Check sheet for the modelled part. Datum: model origin and axes. Units: mm. Face numbers are marked on the shaded views. A direction names the side the tool comes from. Give positions to 0.01 mm unless a question says otherwise; leave off trailing zeros. Write each loop counter-clockwise with the first axis right and the second up, starting at its lowest first coordinate (ties: lowest second). Pieces come first, ordered by that corner, then holes. Notation, with made-up numbers: M 19,72.25 L 48,72.25 A25 cw 48,111.25 Z; hole C 14,-39 d3. An arc over 180 degrees is marked long. Write item = value, one per line. Start each with the question number.
1) Sectioned sample at B-B, the plane y = -51. Record the cut outline in (x, z).
2) Draft check along Y on the marked faces 1 and 2. Enter one of: pulls with the +Y half, pulls with the -Y half, needs draft (parallel to the pull), parting line crosses it, or undercut.
3) Sectioned sample at C-C, the plane y = 81. Record the cut outline in (x, z).
4) Gauge pin test, flat ends, axial feed: pin 1 (1 mm diameter, centred on x = -19, y = 30.5, fed in from +Z); pin 2 (12 mm diameter, centred on x = 21, y = -12, fed in from -Z); pin 3 (12 mm diameter, centred on y = -19, z = -71, fed in from +X). Record the tip position at first contact, or that the pin passes through.
5) Sectioned sample at A-A, the plane z = -68.5. Count the separate pieces of the cut face and the enclosed holes in it, then the cut area to 3 significant figures.
6) Set-up check for the marked faces 3 and 4: record each of +Z, -Z, +X, -X, +Y, -Y from which the full face is reachable in a straight line by a thin tool's end or side.
7) Scan lines: L1, parallel to Y at x = 41, z = 67; L2, parallel to Z at x = -11.5, y = 40.5; L3, parallel to Z at x = 9.5, y = -38.5. Record each from-to range of solid material in increasing order.
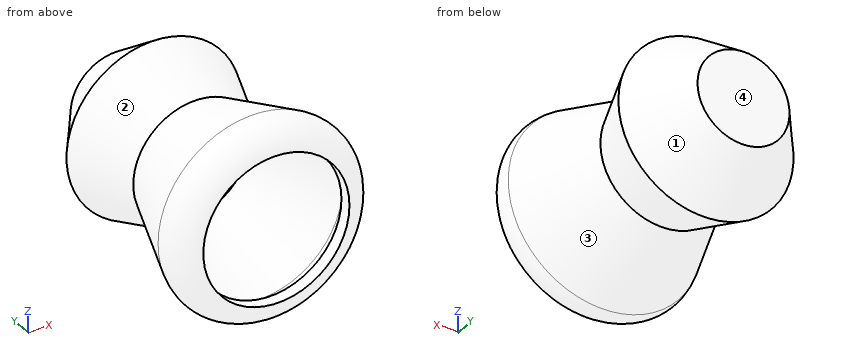
from build123d import *

# Parameters (mm, degrees)
F0_R     = 63.5
F1_DEPTH = 127
F1_TAPER = -20
F2_R     = 25.4
F3_SIZE  = 63.5
F4_T     = -12.7


# Not quite as in the source:
# - a shell that OpenCascade refuses in one call is made with other operations: the cavity is built on its own and cut out


with BuildPart() as f1:
    # F0 (on Front) → F1 (new body, symmetric)
    with BuildSketch(Plane.XZ):
        with Locations((0.2353243763, -0.2353235031)):
            Circle(F0_R)
    extrude(amount=F1_DEPTH, both=True, taper=F1_TAPER)

    # F2
    f2_edges = [f1.edges().sort_by_distance(p)[0] for p in [
        (-109.488895, -127, -0.235324),
    ]]
    fillet(f2_edges, radius=F2_R)

    # F3
    f3_edges = [f1.edges().sort_by_distance(p)[0] for p in [
        (-109.488895, 127, -0.235324),
    ]]
    chamfer(f3_edges, length=F3_SIZE)

    # F4: a shell. OpenCascade refuses it in one call, so the cavity is built on its own and cut out:
    # the body offset inwards by the wall thickness, plus a prism from it out through each open face.
    f4_core = offset(f1.part, amount=F4_T, kind=Kind.INTERSECTION, mode=Mode.PRIVATE)
    f4_exits = [f4_core.faces().sort_by_distance(p)[0] for p in [
        (0.235324, -114.3, -0.235324),
    ]]
    add(f4_core, mode=Mode.SUBTRACT)
    extrude(f4_exits, amount=-F4_T, mode=Mode.SUBTRACT)


solid = f1.part
Data:
q1.outline = C 0.24,-0.24 d164.12; hole C 0.24,-0.24 d137.09
q2.face_1 = pulls with the +Y half
q2.face_2 = undercut
q3.outline = C 0.24,-0.24 d156.87; hole C 0.24,-0.24 d125.86
q4.pin_1 = 72.07
q4.pin_2 = -67.7
q4.pin_3 = 28.92
q5.separate_pieces = 2
q5.enclosed_holes = 1
q5.area = 11,200 mm2
q6.face_3 = none
q6.face_4 = +Z, -Z, +X, -X, +Y
q7.L1 = -126.47 to -113.2, -78.7 to -41.56, 41.56 to 80.72
q7.L2 = -77.59 to -63.89, 63.42 to 77.12
q7.L3 = -77.19 to -63.56, 63.09 to 76.72
